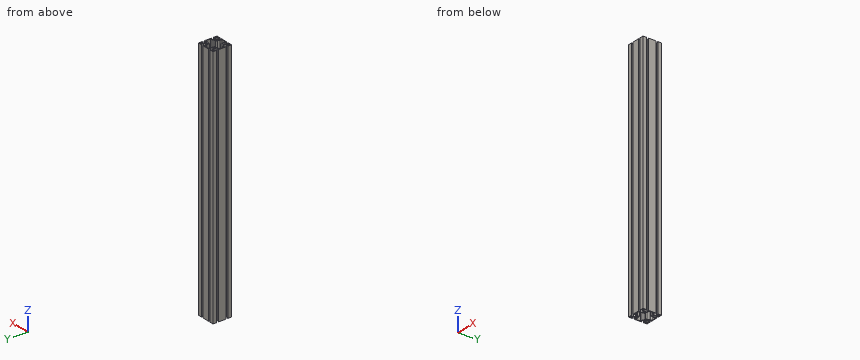
```python
from build123d import *

# Parameters (mm, degrees)
F0_R     = 3
F0_R_2   = 2.5
F1_DEPTH = 787
F2_R     = 2
F3_R     = 7


# Not quite as in the source:
# - a feature names something its author has since deleted; it is built from what else it names


with BuildPart() as f1:
    # F0 (on Top) → F1 (new body)
    with BuildSketch(Plane.XY):
        with BuildLine():
            Line((18.15, -30), (30, -30))
            Line((30, -30), (30, -18.15))
            Line((30, -18.15), (27.5, -18.15))
            Line((27.5, -18.15), (27.5, -20.15))
            Line((27.5, -20.15), (21.5477069044, -20.15))
            ThreePointArc((21.5477069044, -20.15), (19.5, -15), (21.5477069044, -9.85))
            Line((21.5477069044, -9.85), (27.5, -9.85))
            Line((27.5, -9.85), (27.5, -11.85))
            Line((27.5, -11.85), (30, -11.85))
            Line((30, -11.85), (30, 11.85))
            Line((30, 11.85), (27.5, 11.85))
            Line((27.5, 11.85), (27.5, 9.85))
            Line((27.5, 9.85), (21.5477069044, 9.85))
            ThreePointArc((21.5477069044, 9.85), (19.5, 15), (21.5477069044, 20.15))
            Line((21.5477069044, 20.15), (27.5, 20.15))
            Line((27.5, 20.15), (27.5, 18.15))
            Line((27.5, 18.15), (30, 18.15))
            Line((30, 18.15), (30, 30))
            Line((30, 30), (18.15, 30))
            Line((18.15, 30), (18.15, 27.5))
            Line((18.15, 27.5), (20.15, 27.5))
            Line((20.15, 27.5), (20.15, 21.5477069044))
            ThreePointArc((20.15, 21.5477069044), (15, 19.5), (9.85, 21.5477069044))
            Line((9.85, 21.5477069044), (9.85, 27.5))
            Line((9.85, 27.5), (11.85, 27.5))
            Line((11.85, 27.5), (11.85, 30))
            Line((11.85, 30), (-11.85, 30))
            Line((-11.85, 30), (-11.85, 27.5))
            Line((-11.85, 27.5), (-9.85, 27.5))
            Line((-9.85, 27.5), (-9.85, 21.5477069044))
            ThreePointArc((-9.85, 21.5477069044), (-15, 19.5), (-20.15, 21.5477069044))
            Line((-20.15, 21.5477069044), (-20.15, 27.5))
            Line((-20.15, 27.5), (-18.15, 27.5))
            Line((-18.15, 27.5), (-18.15, 30))
            Line((-18.15, 30), (-30, 30))
            Line((-30, 30), (-30, 18.15))
            Line((-30, 18.15), (-27.5, 18.15))
            Line((-27.5, 18.15), (-27.5, 20.15))
            Line((-27.5, 20.15), (-21.5477069044, 20.15))
            ThreePointArc((-21.5477069044, 20.15), (-19.5, 15), (-21.5477069044, 9.85))
            Line((-21.5477069044, 9.85), (-27.5, 9.85))
            Line((-27.5, 9.85), (-27.5, 11.85))
            Line((-27.5, 11.85), (-30, 11.85))
            Line((-30, 11.85), (-30, -11.85))
            Line((-30, -11.85), (-27.5, -11.85))
            Line((-27.5, -11.85), (-27.5, -9.85))
            Line((-27.5, -9.85), (-21.5477069044, -9.85))
            ThreePointArc((-21.5477069044, -9.85), (-19.5, -15), (-21.5477069044, -20.15))
            Line((-21.5477069044, -20.15), (-27.5, -20.15))
            Line((-27.5, -20.15), (-27.5, -18.15))
            Line((-27.5, -18.15), (-30, -18.15))
            Line((-30, -18.15), (-30, -30))
            Line((-30, -30), (-18.15, -30))
            Line((-18.15, -30), (-18.15, -27.5))
            Line((-18.15, -27.5), (-20.15, -27.5))
            Line((-20.15, -27.5), (-20.15, -21.5477069044))
            ThreePointArc((-20.15, -21.5477069044), (-15, -19.5), (-9.85, -21.5477069044))
            Line((-9.85, -21.5477069044), (-9.85, -27.5))
            Line((-9.85, -27.5), (-11.85, -27.5))
            Line((-11.85, -27.5), (-11.85, -30))
            Line((-11.85, -30), (11.85, -30))
            Line((11.85, -30), (11.85, -27.5))
            Line((11.85, -27.5), (9.85, -27.5))
            Line((9.85, -27.5), (9.85, -21.5477069044))
            ThreePointArc((9.85, -21.5477069044), (15, -19.5), (20.15, -21.5477069044))
            Line((20.15, -21.5477069044), (20.15, -27.5))
            Line((20.15, -27.5), (18.15, -27.5))
            Line((18.15, -27.5), (18.15, -30))
        make_face()
        with Locations((-25, -25)):
            Circle(F0_R, mode=Mode.SUBTRACT)
        with Locations((-15, -15)):
            Circle(F0_R_2, mode=Mode.SUBTRACT)
        with Locations((25, -25)):
            Circle(F0_R, mode=Mode.SUBTRACT)
        with Locations((15, -15)):
            Circle(F0_R_2, mode=Mode.SUBTRACT)
        with Locations((-25, 25)):
            Circle(F0_R, mode=Mode.SUBTRACT)
        with Locations((-15, 15)):
            Circle(F0_R_2, mode=Mode.SUBTRACT)
        Polygon((-7, 22), (-7, 27.5), (0, 27.5), (7, 27.5), (7, 22), (10, 16), (10, 10), (16, 10), (22, 7), (27.5, 7), (27.5, 0), (27.5, -7), (22, -7), (16, -10), (10, -10), (10, -16), (7, -22), (7, -27.5), (0, -27.5), (-7, -27.5), (-7, -22), (-10, -16), (-10, -10), (-16, -10), (-22, -7), (-27.5, -7), (-27.5, 0), (-27.5, 7), (-22, 7), (-16, 10), (-10, 10), (-10, 16), align=None, mode=Mode.SUBTRACT)
        with Locations((15, 15)):
            Circle(F0_R_2, mode=Mode.SUBTRACT)
        with Locations((25, 25)):
            Circle(F0_R, mode=Mode.SUBTRACT)
    extrude(amount=F1_DEPTH)

    # F2
    f2_edges = [f1.edges().sort_by_distance(p)[0] for p in [
        (-7, 27.5, 393.5),
        (7, 27.5, 393.5),
    ]]
    fillet(f2_edges, radius=F2_R)

    # F3
    f3_edges = [f1.edges().sort_by_distance(p)[0] for p in [
        (-10, 16, 393.5),
        (10, 16, 393.5),
    ]]
    fillet(f3_edges, radius=F3_R)


solid = f1.part
```
For this review, take the finished solid that the model builds, in its own axes (mm). Round coordinates to 2 decimals unless told otherwise and drop trailing zeros. One line per item, written item: value. Start each with the question number.
(1) Wall thickness on line 1 (Y direction, x = -25, z = 403.5); line 2 (Y direction, x = -15, z = 556); line 3 (Y direction, x = -15.5, z = 578): over which ranges is each line inside the solid? List them lowest first.
(2) We need section A-A (z = 291). Count the separate pieces of the cut face and the enclosed holes in it, and give its area (3 significant figures).
(3) Insertion check: pin 1 (3 mm diameter, centred on y = -14, z = 454, fed in from +X); pin 2 (1 mm diameter, centred on x = -14.5, z = 564.5, fed in from +Y). Each pin has a flat end and moves straight along its axis. Give the tip position at first contact, or say it passes through.
Result:
1. line 1: -30 to -28, -22 to -20.15, -9.85 to -7, 7 to 9.85, 20.15 to 22, 28 to 30
1. line 2: -19.5 to -17.5, -12.5 to -10, 10 to 12.5, 17.5 to 19.5
1. line 3: -19.52 to -17.45, -12.55 to -10, 10 to 12.55, 17.45 to 19.52
2. separate pieces: 1
2. enclosed holes: 9
2. area: 1,080 mm²
3. pin 1: x = 19.93
3. pin 2: y = 19.57
